Source: CAD feature listing. Evaluate the final solid. Frame: model axes, mm. Round coordinates to 2 decimals unless told otherwise and drop trailing zeros. Write each loop counter-clockwise with the first axis right and the second up, starting at its lowest first coordinate (ties: lowest second). Pieces come first, ordered by that corner, then holes.
```python
from build123d import *

# Parameters (mm, degrees)
F0_W     = 127
F0_H     = 76.2
F0_R     = 6.35
F1_DEPTH = 50.8
F2_R     = 12.7
F3_DEPTH = 60.452
F4_R     = 12.7
F5_R     = 12.7
F6_R     = 12.7
F7_R     = 12.7
F8_SIZE  = 6.35
F9_SIZE  = 6.35


with BuildPart() as f1:
    # F0 (on Front) → F1 (new body)
    with BuildSketch(Plane.XZ):
        with Locations((-1.246627, -5.986213)):
            Rectangle(F0_W, F0_H)
        with Locations((-45.696627, -18.686213)):
            Circle(F0_R, mode=Mode.SUBTRACT)
        with Locations((43.203373, 6.713787)):
            Circle(F0_R, mode=Mode.SUBTRACT)
    extrude(amount=F1_DEPTH)

    # F2 (on face) → F3 (cut)
    with BuildSketch(Plane.XZ.offset(50.8)):
        with Locations((-5.936226, -14.195322)):
            Circle(F2_R)
    extrude(amount=-F3_DEPTH, mode=Mode.SUBTRACT)

    # F4
    f4_edges = [f1.edges().sort_by_distance(p)[0] for p in [
        (-64.746627, -25.4, 32.113787),
    ]]
    fillet(f4_edges, radius=F4_R)

    # F5
    f5_edges = [f1.edges().sort_by_distance(p)[0] for p in [
        (62.253373, -25.4, 32.113787),
    ]]
    fillet(f5_edges, radius=F5_R)

    # F6
    f6_edges = [f1.edges().sort_by_distance(p)[0] for p in [
        (62.253373, -25.4, -44.086213),
    ]]
    fillet(f6_edges, radius=F6_R)

    # F7
    f7_edges = [f1.edges().sort_by_distance(p)[0] for p in [
        (-64.746627, -25.4, -44.086213),
    ]]
    fillet(f7_edges, radius=F7_R)

    # F8
    f8_edges = [f1.edges().sort_by_distance(p)[0] for p in [
        (-1.246627, 0, 32.113787),
    ]]
    chamfer(f8_edges, length=F8_SIZE)

    # F9
    f9_edges = [f1.edges().sort_by_distance(p)[0] for p in [
        (-1.246627, -50.8, 32.113787),
    ]]
    chamfer(f9_edges, length=F9_SIZE)


solid = f1.part
```
Q1. Section query B-B, the plane z = 4. Output: boundary loops of the cut face in (x, y), and give its area (3 significant figures).
Q2. Section query C-C, the plane y = -14. Output: boundary loops of the cut face in (x, z).
Q3. Section query A-A, the plane x = -31. Output: boundary loops of the cut face in (y, z).
Q4. Line query: line 1 (X direction, y = -41, z = -23); line 2 (X direction, y = -24.5, z = 6.5); line 3 (X direction, y = -41.5, z = 5). Output: solid intervals per line, ascending.
Q5. Section query D-D, the plane x = 0. Output: boundary loops of the cut face in (y, z).
Q6. Mould query, pull axis X, two halves, no side actions, for faces 1 (the face through (-58.319, -48.375, 25.55)), 2 (the face through (-8.689, -25.756, -26.593)), 3 (the face through (-2, 0, 2)), 4 (the face through (55.75, -2.51, 25.75)). Classes: pulls with the +X half, pulls with the -X half, needs draft (parallel to the pull), parting line crosses it, or undercut.
Filled in:
1. outline: (-64.75, -44.45) - (-58.4, -50.8) - (37.46, -50.8) - (37.46, 0) - (-58.4, 0) - (-64.75, -6.35) - close; (48.94, -50.8) - (55.9, -50.8) - (62.25, -44.45) - (62.25, -6.35) - (55.9, 0) - (48.94, 0) - close
1. area: 5,790 mm2
2. outline: (-64.75, -31.39) arc R12.7 ccw to (-52.05, -44.09) - (49.55, -44.09) arc R12.7 ccw to (62.25, -31.39) - (62.25, 19.41) arc R12.7 ccw to (49.55, 32.11) - (-52.05, 32.11) arc R12.7 ccw to (-64.75, 19.41) - close; hole circle Ø12.7 at (-45.7, -18.69); hole circle Ø25.4 at (-5.94, -14.2); hole circle Ø12.7 at (43.2, 6.71)
3. outline: (-50.8, -37.74) - (-44.45, -44.09) - (-6.35, -44.09) - (0, -37.74) - (0, 25.76) - (-6.35, 32.11) - (-44.45, 32.11) - (-50.8, 25.76) - close
4. line 1: x = -64.75 to -50.36, -41.04 to -15.09, 3.22 to 62.25
4. line 2: x = -64.75 to 36.86, 49.55 to 62.25
4. line 3: x = -64.75 to 37.09, 49.32 to 62.25
5. outline: (-50.8, -37.74) - (-44.45, -44.09) - (-6.35, -44.09) - (0, -37.74) - (0, -25.42) - (-50.8, -25.42) - close; (-50.8, -2.97) - (0, -2.97) - (0, 25.76) - (-6.35, 32.11) - (-44.45, 32.11) - (-50.8, 25.76) - close
6. face 1: pulls with the -X half
6. face 2: undercut
6. face 3: needs draft
6. face 4: pulls with the +X half
